Design review of the part built by this model. Coordinates are the model's own, in mm. A direction names the side the tool comes from. Coordinates: 2 decimals unless noted, no trailing zeros. Write each loop counter-clockwise with the first axis right and the second up, starting at its lowest first coordinate (ties: lowest second). Pieces come first, ordered by that corner, then holes.
Q1. Machinability: for faces 3 (the flat face through (30, 43, -43)), 4 (the cylindrical face through (-50.28, -16.39, 52.06)), 5 (the flat face through (-70, 11, -1)), which of the approach directions +Z, -Z, +X, -X, +Y, -Y give a long, thin tool a straight path to every point of the face, cutting with its end or side? Answer none if there is none.
Q2. Mouldability with a two-part tool opening along Z and no side actions: class faces 1 (the cylindrical face through (0.98, -8.508, -1.117)), 2 (the flat face through (70, 11, 1)) as pulls with the +Z half, pulls with the -Z half, needs draft (parallel to the pull), parting line crosses it, or undercut.
Q3. For probe 1 along Z at (x, y) = (-43, -40); probe 2 along X at (y, z) = (55, -24); probe 3 along Z at (x, y) = (-20.5, 0), list the stretches that pass through material, from the lowest coordinate up.
Q4. Insertion check: pin 1 (8 mm diameter, centred on x = 27, y = 78.5, fed in from -Z); pin 2 (4 mm diameter, centred on x = -13, z = 9.5, fed in from -Y); pin 3 (22.5 mm diameter, centred on y = 0, z = 0, fed in from +X); pin 4 (8 mm diameter, centred on x = -35.5, y = -27, fed in from -Z). Each pin has a flat end and moves straight along its axis. Give the tip position at first contact, or say it passes through.
Q5. Take a section at A-A (x = 11). Give the boundary of the cut face in (y, z), and give its area (3 significant figures).
```python
from build123d import *

# Parameters (mm, degrees)
F3_DEPTH = 25


with BuildPart() as f1:
    # F0 (on Front) → F1 (revolve)
    with BuildSketch(Plane.XZ):
        with BuildLine():
            Line((-70, 54.58075), (-70, 8.58075))
            Line((-70, 8.58075), (70, 8.58075))
            Line((70, 8.58075), (70, 54.58075))
            Line((70, 54.58075), (30, 54.58075))
            Line((30, 54.58075), (30, 208.038476))
            ThreePointArc((30, 208.038476), (0, 200), (-30, 208.038476))
            Line((-30, 208.038476), (-30, 54.58075))
            Line((-30, 54.58075), (-70, 54.58075))
        make_face()
        with BuildLine():
            ThreePointArc((60, 260), (-30, 311.961524), (-30, 208.038476))
            ThreePointArc((-30, 208.038476), (0, 200), (30, 208.038476))
            ThreePointArc((30, 208.038476), (51.961524, 230), (60, 260))
        make_face()
    revolve(axis=Axis((0, 0, 0), (1, 0, 0)))

    # F2 (on face) → F3 (join)
    with BuildSketch(Plane(origin=(-30, 0, 0), x_dir=(0, -1, 0), z_dir=(-1, 0, 0))):
        with BuildLine():
            ThreePointArc((-55.462766, 188.029161), (-61.774314, 182.493227), (-61.643278, 174.098882))
            Line((-61.643278, 174.098882), (-12.55207, 72.159939))
            ThreePointArc((-12.55207, 72.159939), (-8.665392, 67.910717), (-3.079813, 66.509481))
            ThreePointArc((-3.079813, 66.509481), (0, 66.58075), (3.079813, 66.509481))
            ThreePointArc((3.079813, 66.509481), (8.665392, 67.910717), (12.55207, 72.159939))
            Line((12.55207, 72.159939), (61.643278, 174.098882))
            ThreePointArc((61.643278, 174.098882), (61.774314, 182.493227), (55.462766, 188.029161))
            ThreePointArc((55.462766, 188.029161), (0, 196.038476), (-55.462766, 188.029161))
        make_face()
    extrude(amount=-F3_DEPTH)


solid = f1.part
```
Response:
1. face 3: +X
1. face 4: -X
1. face 5: +Z, -Z, -X, +Y, -Y
2. face 1: undercut
2. face 2: needs draft
3. probe 1: z = -299.18 to -214.46, -37.14 to 37.14, 214.46 to 299.18
3. probe 2: x = -30 to 30
3. probe 3: z = -316.39 to -8.58, 8.58 to 316.39
4. pin 1: stops at z = -305.77
4. pin 2: stops at y = -318.85
4. pin 3: stops at x = 70
4. pin 4: stops at z = -309.92
5. outline: circle Ø637.97 at (0, 0); hole circle Ø17.16 at (0, 0)
5. area: 319,000 mm2
